Work out the finished part from the listing and answer in its coordinate system (mm). A direction names the side the tool comes from. Round coordinates to 2 decimals unless told otherwise and drop trailing zeros. Order: outer loops, then holes, each group sorted by start corner. A loop starts at its lowest first (then second) coordinate and runs counter-clockwise, first axis right, second up. Notation, with made-up numbers: (85, 42.5) - (99, 42.5) arc R38 cw to (99, 80.5) - close; hole circle Ø2 at (49, 55). An arc over 180 degrees is marked (long way). Answer in a Markdown table with one row per item.
from build123d import *

# Parameters (mm, degrees)
BOSS_EXTRUDE1_DEPTH = 7
SKETCH2_W           = 4
SKETCH2_H           = 35
SKETCH3_W           = 1
SKETCH3_H           = 21
FILLET1_R           = 1
SKETCH6_OUTSIDE_W   = 78.792
SKETCH6_OUTSIDE_H   = 76.626
SKETCH6_OUTSIDE_R   = 7
CUT_EXTRUDE1_DEPTH  = 44.339743116
CUT_EXTRUDE1_DRAFT  = -30


with BuildPart() as part:
    # Sketch1 → Boss-Extrude1 (new body)
    with BuildSketch(Plane.XY):
        Polygon((4.041451884, 7), (-4.041451884, 7), (-8.082903769, 0), (-4.041451884, -7), (4.041451884, -7), (8.082903769, 0), align=None)
    extrude(amount=BOSS_EXTRUDE1_DEPTH)

    # Sketch2 → Revolve1 (revolve)
    with BuildSketch(Plane(origin=(0, 0, 0), x_dir=(1, 0, 0), z_dir=(0, 1, 0))):
        with Locations((-2, -24.5)):
            Rectangle(SKETCH2_W, SKETCH2_H)
    revolve(axis=Axis((0, 0, -34.920005339), (0, 0, 1)))

    # Sketch3 → Cut-Revolve1 (revolve, cut)
    with BuildSketch(Plane(origin=(0, 0, 0), x_dir=(1, 0, 0), z_dir=(0, 1, 0))):
        with Locations((-3.5, -17.5)):
            Rectangle(SKETCH3_W, SKETCH3_H)
    revolve(axis=Axis((0, 0, -11.162931032), (0, 0, 1)), mode=Mode.SUBTRACT)

    # Sketch5 → Cut-Revolve11 (revolve, cut)
    with BuildSketch(Plane(origin=(0, 0, 0), x_dir=(1, 0, 0), z_dir=(0, 1, 0))):
        Polygon((-5e-05, -42), (-4, -38.00005), (-4, -42), align=None)
    revolve(axis=Axis((0, 0, -15.823423108), (0, 0, 1)), mode=Mode.SUBTRACT)

    # Fillet1
    fillet1_edges = [part.edges().sort_by_distance(p)[0] for p in [
        (3, 0, 28),
        (3, 0, 7),
    ]]
    fillet(fillet1_edges, radius=FILLET1_R - 0.0001)  # a hair under: the kernel refuses the full size


with BuildPart() as cut_extrude1_tool:
    # Sketch6 outside → Cut-Extrude1 (with draft: the straight prism first)
    with BuildSketch(Plane(origin=(0, 0, 0), x_dir=(-1, 0, 0), z_dir=(0, 0, -1))):
        Rectangle(SKETCH6_OUTSIDE_W, SKETCH6_OUTSIDE_H)
        Circle(SKETCH6_OUTSIDE_R, mode=Mode.SUBTRACT)
    extrude(amount=-CUT_EXTRUDE1_DEPTH)
    # Cut-Extrude1: the draft: its side faces are tilted about the plane it starts from
    cut_extrude1_sides = [cut_extrude1_tool.faces().sort_by_distance(p)[0] for p in [
        (0, -38.313, 22.169871558),
        (-39.396, 0, 22.169871558),
        (0, 38.313, 22.169871558),
        (39.396, 0, 22.169871558),
        (7, 0, 22.169871558),
    ]]
    draft(cut_extrude1_sides, Plane(origin=(0, 0, 0), x_dir=(-1, 0, 0), z_dir=(0, 0, -1)), CUT_EXTRUDE1_DRAFT)


with BuildPart() as part_1:
    add(part.part)

    # Cut-Extrude1: cut by cut_extrude1_tool
    add(cut_extrude1_tool.part, mode=Mode.SUBTRACT)


solid = part_1.part
1) Which of the six approach directions +Z, -Z, +X, -X, +Y, -Y give full straight-line access (tool end or side, diameter ignored) to faces 4 (the face through (0.867, 3.905, 32.93)), 5 (the face through (6.09, 3.45, 3.45))?
Filled in:
| item | result |
|---|---|
| face 4 | +Z |
| face 5 | +Z, -Z, +X, +Y |
2) Each of these flat-tipped pins is pushed along its axis until it touches: pin 1 (6 mm diameter, centred on x = 5, z = 30, fed in from +Y); pin 2 (4 mm diameter, centred on x = 3, z = 24, fed in from +Y); pin 3 (8 mm diameter, centred on y = -4.5, z = 37.5, fed in from +X). Where does it stop, or does it pass through?
Filled in:
| item | result |
|---|---|
| pin 1 | stops at y = 3.46 |
| pin 2 | stops at y = 2.83 |
| pin 3 | stops at x = 3.97 |
3) The mould has two halves that part along Z. Classify faces 1 (the face through (3, 0, 17)), 2 (the face through (0, 7, 3)), 3 (the face through (3.614, 6.295, 0.447)): released by +Z, released by -Z, zero draft, split by the parting line, or undercut.
Filled in:
| item | result |
|---|---|
| face 1 | undercut |
| face 2 | zero draft |
| face 3 | released by -Z |
4) Find the intervals of material crossed by probe 1 along Z at (x, y) = (-5, 3); probe 2 along Z at (x, y) = (-1.25, -3.5); probe 3 along Z at (x, y) = (2.5, 3), in increasing order. Write a range as from..to.
Filled in:
| item | result |
|---|---|
| probe 1 | z = 0..7 |
| probe 2 | z = 0..7.04, 27.96..38.28 |
| probe 3 | z = 0..7, 28..38.09 |
5) Find section B-B, the plane z = 13. Give the vertices of the cut face in (x, y).
Filled in:
| item | result |
|---|---|
| outline | circle Ø6 at (0, 0) |
6) Find section C-C, the plane z = 31. Give the vertices of the cut face in (x, y), then the cut area to 3 significant figures.
Filled in:
| item | result |
|---|---|
| outline | circle Ø8 at (0, 0) |
| area | 50.3 mm^2 |
7) Find section A-A, the plane z = 4. Give the vertices of the cut face in (x, y), then the cut area to 3 significant figures.
Filled in:
| item | result |
|---|---|
| outline | (-8.08, 0) - (-4.04, -7) - (4.04, -7) - (8.08, 0) - (4.04, 7) - (-4.04, 7) - close |
| area | 170 mm^2 |
